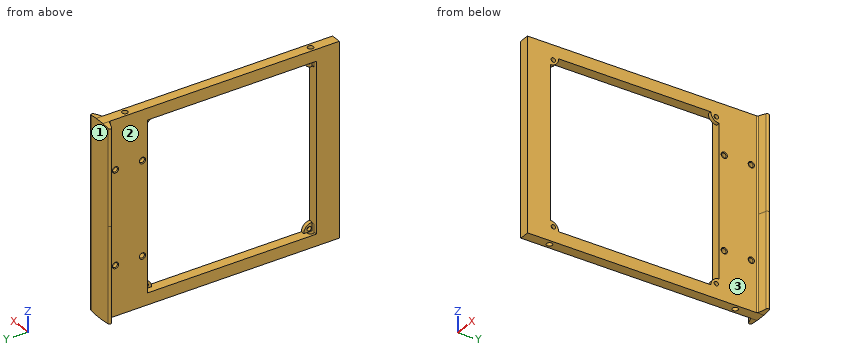
from build123d import *
from build123d.topology import SkipClean

# Parameters (mm, degrees)
BOSS_EXTRUDE1_DEPTH                  = 70
M4_TAPPED_HOLE1_D                    = 3.3
M4_TAPPED_HOLE1_DEPTH                = 11.5
M4_TAPPED_HOLE1_TIP                  = 0.991420021
M4_TAPPED_HOLE1_ON_FACE_2_D          = 3.3
M4_TAPPED_HOLE1_ON_FACE_2_DEPTH      = 11.5
M4_TAPPED_HOLE1_ON_FACE_2_TIP        = 0.991420021
BOSS_EXTRUDE3_REACH                  = 92.322
BOSS_EXTRUDE3_END_RADIUS             = 57
BOSS_EXTRUDE3_DIRECTION_2_REACH      = 92.322
BOSS_EXTRUDE3_DIRECTION_2_END_RADIUS = 57
CUT_EXTRUDE4_DEPTH                   = 91.671109116
CUT_EXTRUDE4_DEPTH_BACK              = 91.671109116
SKETCH5_W                            = 100
SKETCH5_H                            = 100
BOSS_EXTRUDE4_START                  = 0.8
SKETCH6_R                            = 1.27
BOSS_EXTRUDE4_DEPTH                  = 2.2
SKETCH12_R                           = 1.84
CUT_EXTRUDE6_DEPTH                   = 2.58


# Read off the part's stored shape, not the designer's step: Hole1
with BuildPart() as part:
    # Sketch1 → Boss-Extrude1 (new, symmetric)
    with BuildSketch(Plane(origin=(0, 0, 0), x_dir=(1, 0, 0), z_dir=(0, 1, 0))):
        with BuildLine():
            Line((-3, 56.920997883), (-3, -56.920997883))
            ThreePointArc((-3, -56.920997883), (0, -57), (3, -56.920997883))
            Line((3, -56.920997883), (3, 56.920997883))
            ThreePointArc((3, 56.920997883), (0, 57), (-3, 56.920997883))
        make_face()
    extrude(amount=BOSS_EXTRUDE1_DEPTH, both=True)

    # M4 Tapped Hole1
    with Locations(Plane(origin=(0, 55, 57), x_dir=(1, 0, 0), z_dir=(0, 0, 1))):
        with Locations((0, 0), (0, -110)):
            Hole(M4_TAPPED_HOLE1_D / 2, depth=M4_TAPPED_HOLE1_DEPTH)
            with Locations((0, 0, -(M4_TAPPED_HOLE1_DEPTH + M4_TAPPED_HOLE1_TIP / 2))):  # 118° drill point
                Cone(0, M4_TAPPED_HOLE1_D / 2, M4_TAPPED_HOLE1_TIP, mode=Mode.SUBTRACT)

    # M4 Tapped Hole1 on face 2
    with Locations(Plane(origin=(0, 55, -57), x_dir=(-1, 0, 0), z_dir=(0, 0, -1))):
        with Locations((0, 0), (0, -110)):
            Hole(M4_TAPPED_HOLE1_ON_FACE_2_D / 2, depth=M4_TAPPED_HOLE1_ON_FACE_2_DEPTH)
            with Locations((0, 0, -(M4_TAPPED_HOLE1_ON_FACE_2_DEPTH + M4_TAPPED_HOLE1_ON_FACE_2_TIP / 2))):  # 118° drill point
                Cone(0, M4_TAPPED_HOLE1_ON_FACE_2_D / 2, M4_TAPPED_HOLE1_ON_FACE_2_TIP, mode=Mode.SUBTRACT)

    # Boss-Extrude3: up to this cylinder (the profile starts inside it)
    with SkipClean():  # the faces are left unmerged after this step: merging them gives an invalid solid
        boss_extrude3_end = Plane(origin=(0, 67.695148, 0), z_dir=(0, -1, 0)) * Cylinder(BOSS_EXTRUDE3_END_RADIUS, 299.644, mode=Mode.PRIVATE)
        # Sketch4 → Boss-Extrude3 (add, up to the surface)
        with BuildSketch(Plane.XY, mode=Mode.PRIVATE) as boss_extrude3_sk1:
            with BuildLine():
                Line((-7.5, 70), (7.5, 70))
                ThreePointArc((7.5, 70), (8.48399318, 69.178206122), (7.850707217, 68.063514844))
                Line((7.850707217, 68.063514844), (3.649292783, 66.490114182))
                ThreePointArc((3.649292783, 66.490114182), (3.178200993, 66.123406518), (3, 65.553629026))
                Line((3, 65.553629026), (3, 64))
                Line((3, 64), (-3, 64))
                Line((-3, 64), (-3, 65.553629026))
                ThreePointArc((-3, 65.553629026), (-3.178200993, 66.123406518), (-3.649292783, 66.490114182))
                Line((-3.649292783, 66.490114182), (-7.850707217, 68.063514844))
                ThreePointArc((-7.850707217, 68.063514844), (-8.48399318, 69.178206122), (-7.5, 70))
            make_face()
        boss_extrude3_tool1 = extrude(boss_extrude3_sk1.sketch, amount=BOSS_EXTRUDE3_REACH, mode=Mode.PRIVATE) & boss_extrude3_end
        add(boss_extrude3_tool1.solids().sort_by_distance((0, 67.695148, 0))[0])

    # Boss-Extrude3 direction 2: up to this cylinder (the profile starts inside it)
    with SkipClean():  # the faces are left unmerged after this step: merging them gives an invalid solid
        boss_extrude3_direction_2_end = Plane(origin=(0, 67.695148, 0), z_dir=(0, -1, 0)) * Cylinder(BOSS_EXTRUDE3_DIRECTION_2_END_RADIUS, 299.644, mode=Mode.PRIVATE)
        # Sketch4 → Boss-Extrude3 direction 2 (add, up to the surface)
        with BuildSketch(Plane.XY, mode=Mode.PRIVATE) as boss_extrude3_direction_2_sk1:
            with BuildLine():
                Line((-7.5, 70), (7.5, 70))
                ThreePointArc((7.5, 70), (8.48399318, 69.178206122), (7.850707217, 68.063514844))
                Line((7.850707217, 68.063514844), (3.649292783, 66.490114182))
                ThreePointArc((3.649292783, 66.490114182), (3.178200993, 66.123406518), (3, 65.553629026))
                Line((3, 65.553629026), (3, 64))
                Line((3, 64), (-3, 64))
                Line((-3, 64), (-3, 65.553629026))
                ThreePointArc((-3, 65.553629026), (-3.178200993, 66.123406518), (-3.649292783, 66.490114182))
                Line((-3.649292783, 66.490114182), (-7.850707217, 68.063514844))
                ThreePointArc((-7.850707217, 68.063514844), (-8.48399318, 69.178206122), (-7.5, 70))
            make_face()
        boss_extrude3_direction_2_tool1 = extrude(boss_extrude3_direction_2_sk1.sketch, amount=-BOSS_EXTRUDE3_DIRECTION_2_REACH, mode=Mode.PRIVATE) & boss_extrude3_direction_2_end
        add(boss_extrude3_direction_2_tool1.solids().sort_by_distance((0, 67.695148, 0))[0])

    # Sketch5 → Cut-Extrude4 (cut, two sides: drawn at the far end of the back side and taken through both)
    with SkipClean():  # the faces are left unmerged after this step: merging them gives an invalid solid
        with BuildSketch(Plane(origin=(0, 0, 0), x_dir=(0, 0, -1), z_dir=(1, 0, 0)).offset(-CUT_EXTRUDE4_DEPTH_BACK)):
            with Locations((0, -6.446370974)):
                Rectangle(SKETCH5_W, SKETCH5_H)
        extrude(amount=CUT_EXTRUDE4_DEPTH + CUT_EXTRUDE4_DEPTH_BACK, mode=Mode.SUBTRACT)

    # Sketch6 → Boss-Extrude4 (add)
    # profile 1 of 4: a face of its own
    with SkipClean():  # the faces are left unmerged after this step: merging them gives an invalid solid
        with BuildSketch(Plane(origin=(0, 0, 0), x_dir=(0, 0, -1), z_dir=(1, 0, 0)).offset(BOSS_EXTRUDE4_START)):
            with BuildLine():
                Line((50, 43.553629026), (50, 38.603881557))
                ThreePointArc((50, 38.603881557), (46.5, 40.053629026), (45.050252532, 43.553629026))
                Line((45.050252532, 43.553629026), (50, 43.553629026))
            make_face()
            with Locations(Location((48.25, 41.803629026, 0), (0, 0, 180))):
                Circle(SKETCH6_R, mode=Mode.SUBTRACT)
        # profile 2 of 4: a face of its own
        with BuildSketch(Plane(origin=(0, 0, 0), x_dir=(0, 0, -1), z_dir=(1, 0, 0)).offset(BOSS_EXTRUDE4_START)):
            with BuildLine():
                Line((-50, 43.553629026), (-45.050252532, 43.553629026))
                ThreePointArc((-45.050252532, 43.553629026), (-46.5, 40.053629026), (-50, 38.603881557))
                Line((-50, 38.603881557), (-50, 43.553629026))
            make_face()
            with Locations(Location((-48.25, 41.803629026, 0), (0, 0, 180))):
                Circle(SKETCH6_R, mode=Mode.SUBTRACT)
        # profile 3 of 4: a face of its own
        with BuildSketch(Plane(origin=(0, 0, 0), x_dir=(0, 0, -1), z_dir=(1, 0, 0)).offset(BOSS_EXTRUDE4_START)):
            with BuildLine():
                Line((-50, -56.446370974), (-50, -51.496623506))
                ThreePointArc((-50, -51.496623506), (-46.5, -52.946370974), (-45.050252532, -56.446370974))
                Line((-45.050252532, -56.446370974), (-50, -56.446370974))
            make_face()
            with Locations(Location((-48.25, -54.696370974, 0), (0, 0, 180))):
                Circle(SKETCH6_R, mode=Mode.SUBTRACT)
        # profile 4 of 4: a face of its own
        with BuildSketch(Plane(origin=(0, 0, 0), x_dir=(0, 0, -1), z_dir=(1, 0, 0)).offset(BOSS_EXTRUDE4_START)):
            with BuildLine():
                Line((50, -56.446370974), (45.050252532, -56.446370974))
                ThreePointArc((45.050252532, -56.446370974), (46.5, -52.946370974), (50, -51.496623506))
                Line((50, -51.496623506), (50, -56.446370974))
            make_face()
            with Locations(Location((48.25, -54.696370974, 0), (0, 0, 180))):
                Circle(SKETCH6_R, mode=Mode.SUBTRACT)
        extrude(amount=BOSS_EXTRUDE4_DEPTH)

    # Hole1 outline → Hole1 (revolve, cut)
    with SkipClean():  # the faces are left unmerged after this step: merging them gives an invalid solid
        with BuildSketch(Plane(origin=(0, 46.553629026, -27.6225), x_dir=(0, 1, 0), z_dir=(0, 0, -1))):
            Polygon((0, -3), (1.42, -3), (1.42, 2.58), (1.84, 3), (0, 3), align=None)
        hole1 = revolve(axis=Axis((0, 46.553629026, -27.6225), (1, 0, 0)), mode=Mode.SUBTRACT)

    # Hole1 2 outline → Hole1 2 (revolve, cut)
    with SkipClean():  # the faces are left unmerged after this step: merging them gives an invalid solid
        with BuildSketch(Plane(origin=(0, 62.553629026, 27.6225), x_dir=(0, 1, 0), z_dir=(0, 0, -1))):
            Polygon((0, -3), (1.42, -3), (1.42, 2.58), (1.84, 3), (0, 3), align=None)
        hole1_2 = revolve(axis=Axis((0, 62.553629026, 27.6225), (1, 0, 0)), mode=Mode.SUBTRACT)

    # Hole1 3 outline → Hole1 3 (revolve, cut)
    with SkipClean():  # the faces are left unmerged after this step: merging them gives an invalid solid
        with BuildSketch(Plane(origin=(0, 46.553629026, 27.6225), x_dir=(0, 1, 0), z_dir=(0, 0, -1))):
            Polygon((0, -3), (1.42, -3), (1.42, 2.58), (1.84, 3), (0, 3), align=None)
        hole1_3 = revolve(axis=Axis((0, 46.553629026, 27.6225), (1, 0, 0)), mode=Mode.SUBTRACT)

    # Hole1 4 outline → Hole1 4 (revolve, cut)
    with SkipClean():  # the faces are left unmerged after this step: merging them gives an invalid solid
        with BuildSketch(Plane(origin=(0, 62.553629026, -27.6225), x_dir=(0, 1, 0), z_dir=(0, 0, -1))):
            Polygon((0, -3), (1.42, -3), (1.42, 2.58), (1.84, 3), (0, 3), align=None)
        hole1_4 = revolve(axis=Axis((0, 62.553629026, -27.6225), (1, 0, 0)), mode=Mode.SUBTRACT)

    # Mirror1: Hole1, Hole1 2, Hole1 3, Hole1 4 across plane
    with SkipClean():  # the faces are left unmerged after this step: merging them gives an invalid solid
        add(hole1.mirror(Plane(origin=(0, 0, 0), x_dir=(0, 0, 1), z_dir=(1, 0, 0))), mode=Mode.SUBTRACT)
        add(hole1_2.mirror(Plane(origin=(0, 0, 0), x_dir=(0, 0, 1), z_dir=(1, 0, 0))), mode=Mode.SUBTRACT)
        add(hole1_3.mirror(Plane(origin=(0, 0, 0), x_dir=(0, 0, 1), z_dir=(1, 0, 0))), mode=Mode.SUBTRACT)
        add(hole1_4.mirror(Plane(origin=(0, 0, 0), x_dir=(0, 0, 1), z_dir=(1, 0, 0))), mode=Mode.SUBTRACT)

    # Sketch12 → Cut-Extrude6 (cut, symmetric)
    with SkipClean():  # the faces are left unmerged after this step: merging them gives an invalid solid
        with BuildSketch(Plane(origin=(0, 0, 0), x_dir=(0, 0, -1), z_dir=(1, 0, 0))):
            with Locations((-27.6225, 62.553629026)):
                Circle(SKETCH12_R)
            with Locations((-27.6225, 46.553629026)):
                Circle(SKETCH12_R)
            with Locations((27.6225, 62.553629026)):
                Circle(SKETCH12_R)
            with Locations((27.6225, 46.553629026)):
                Circle(SKETCH12_R)
        extrude(amount=CUT_EXTRUDE6_DEPTH, both=True, mode=Mode.SUBTRACT)


solid = part.part
The model under review builds one solid part; all positions refer to its coordinate system, in mm. Face numbers are marked on the shaded views. Give positions to 0.01 mm unless a question says otherwise; leave off trailing zeros. Write each loop counter-clockwise with the first axis right and the second up, starting at its lowest first coordinate (ties: lowest second). Pieces come first, ordered by that corner, then holes.
1. For P1, Ø1.5, axis at y = -54.7, z = 48.25, coming from the +X side; P2, Ø0.7, axis at x = 1.5, y = -55, coming from the -Z side; P3, Ø4, axis at y = 46.55, z = -27.62, coming from the +X side; P4, Ø1.1, axis at y = 62.5, z = -26.5, coming from the -X side, all flat-tipped, find the tip position at first contact; note any pin that passes through.
2. Wall thickness on L1, parallel to Y at x = 0, z = 49.5; L2, parallel to Z at x = -0.75, y = -23; L3, parallel to Y at x = -0.5, z = 6: over which ranges is each line inside the solid? List them lowest first.
3. Add section A-A, the plane z = 24. Write out the cut boundary in (x, y).
4. Add section B-B, the plane y = 19. Write out the cut boundary in (x, z), plus the area to 3 significant figures.
5. Draft analysis for pull direction X (two halves, no side actions). For the marked faces 1, 2 and 3, state which applies: +X half, -X half, draft (parallel to the pull), parting line (faces both ways), or undercut.
Worked answers:
1. P1: passes through
1. P2: stops at z = -56.98
1. P3: stops at x = 3
1. P4: stops at x = -2.83
2. L1: y = -70 to -56.65, 43.55 to 53.35, 56.65 to 70
2. L2: z = -57 to -50, 50 to 57
2. L3: y = -70 to -56.45, 43.55 to 70
3. outline: (-7.85, 68.06) - (-3.65, 66.49) arc R1 cw to (-3, 65.55) - (-3, 43.55) - (3, 43.55) - (3, 65.55) arc R1 cw to (3.65, 66.49) - (7.85, 68.06) arc R1 ccw to (7.5, 70) - (-7.5, 70) arc R1 ccw to start; (-3, -70) - (3, -70) - (3, -56.45) - (-3, -56.45) - close
4. outline: (-3, -56.92) arc R57 ccw to (3, -56.92) - (3, -50) - (-3, -50) - close; (-3, 50) - (3, 50) - (3, 56.92) arc R57 ccw to (-3, 56.92) - close
4. area: 83.7 mm2
5. face 1: draft
5. face 2: -X half
5. face 3: +X half
